from build123d import *

# Parameters (mm, degrees)
F1_DEPTH = 6.35
F2_R     = 5.08
F3_R     = 2.54
F4_R     = 2.54


with BuildPart() as f1:
    # F0 (on Top) → F1 (new body)
    with BuildSketch(Plane.XY):
        with BuildLine():
            Line((8.920526, 4.445), (10.377061, 4.445))
            ThreePointArc((10.377061, 4.445), (-11.288995, 0), (10.377061, -4.445))
            Line((10.377061, -4.445), (8.920526, -4.445))
            Line((8.920526, -4.445), (8.920526, 4.445))
        make_face()
        Polygon((3.739498, -6.477), (-3.739498, -6.477), (-7.478995, 0), (-3.739498, 6.477), (3.739498, 6.477), (7.478995, 0), align=None, mode=Mode.SUBTRACT)
        with BuildLine():
            ThreePointArc((10.377061, -4.445), (11.058662, -2.268791), (11.288995, 0))
            ThreePointArc((11.288995, 0), (11.058662, 2.268791), (10.377061, 4.445))
            Line((10.377061, 4.445), (8.920526, 4.445))
            Line((8.920526, 4.445), (8.920526, -4.445))
            Line((8.920526, -4.445), (10.377061, -4.445))
        make_face()
        with BuildLine():
            ThreePointArc((10.377061, 4.445), (11.058662, 2.268791), (11.288995, 0))
            ThreePointArc((11.288995, 0), (11.058662, -2.268791), (10.377061, -4.445))
            Line((10.377061, -4.445), (72.420526, -4.445))
            Line((72.420526, -4.445), (72.420526, 4.445))
            Line((72.420526, 4.445), (10.377061, 4.445))
        make_face()
    extrude(amount=F1_DEPTH)

    # F2
    f2_edges = [f1.edges().sort_by_distance(p)[0] for p in [
        (10.377061, -4.445, 3.175),
        (10.377061, 4.445, 3.175),
    ]]
    fillet(f2_edges, radius=F2_R)

    # F3
    f3_edges = [f1.edges().sort_by_distance(p)[0] for p in [
        (72.420526, 4.445, 3.175),
        (72.420526, -4.445, 3.175),
    ]]
    fillet(f3_edges, radius=F3_R)

    # F4
    f4_edges = [f1.edges().sort_by_distance(p)[0] for p in [
        (41.596433, -4.445, 6.35),
    ]]
    fillet(f4_edges, radius=F4_R)


solid = f1.part
The listing builds one solid part. Answer for the finished solid, in the listing's coordinates (mm). A direction names the side the tool comes from. Coordinates: 2 decimals unless noted, no trailing zeros. Order: outer loops, then holes, each group sorted by start corner. A loop starts at its lowest first (then second) coordinate and runs counter-clockwise, first axis right, second up.
Q1. A cutting plane is placed at B-B, the plane x = 22. Write down the section's boundary in (y, z) (3 decimals).
Q2. Which of the six approach directions +Z, -Z, +X, -X, +Y, -Y give full straight-line access (tool end or side, diameter ignored) to faces 5 (the face through (41.2, 3.721, 5.586)), 6 (the face through (41, -4.445, 2)), 7 (the face through (11, 5, 2)), 8 (the face through (5.583, 3.284, 3.131))?
Q3. A cutting plane is placed at A-A, the plane z = 2. Write down the section's boundary in (x, y) (1 decimal).
Q4. For a pull along X with two mould halves and no side action, classify faces 1 (the face through (41.992, -3.721, 5.586)), 2 (the face through (71.696, 0.027, 5.586)), 3 (the face through (5.635, -3.193, 3.131)), 4 (the face through (-11.28, 0.4, 1.88)) as pulls with the +X half, pulls with the -X half, needs draft (parallel to the pull), parting line crosses it, or undercut.
Q5. Given P1, Ø1.5, axis at x = 51, z = 3.5, coming from the +Y side (3 decimals); P2, Ø3, axis at y = 3.5, z = 5.5, coming from the +X side; P3, Ø12, axis at x = 17, y = 8.5, coming from the +Z side, each flat-ended and moving along its own axis, determine where each tip first touches the part or whether it passes through.
Q6. Consider line 1 (Y direction, x = 39, z = 0.5) (3 decimals); line 2 (X direction, y = 5, z = 2); line 3 (X direction, y = -3, z = 2.75). Determine where each line is inside the solid, lowest interval first.
Answers follow:
1. outline: (-4.445, 0) - (4.445, 0) - (4.445, 3.81) arc R2.54 ccw to (1.905, 6.35) - (-1.905, 6.35) arc R2.54 ccw to (-4.445, 3.81) - close
2. face 5: +Z, +X, +Y
2. face 6: +Z, -Z, +X, -Y
2. face 7: +Z, -Z, +X, +Y
2. face 8: +Z, -Z
3. outline: (9.2, -6.6) arc R5.1 cw to (13.3, -4.4) - (69.9, -4.4) arc R2.5 ccw to (72.4, -1.9) - (72.4, 1.9) arc R2.5 ccw to (69.9, 4.4) - (13.3, 4.4) arc R5.1 cw to (9.2, 6.6) arc R11.3 ccw (long way) to start; hole (-7.5, 0) - (-3.7, -6.5) - (3.7, -6.5) - (7.5, 0) - (3.7, 6.5) - (-3.7, 6.5) - close
4. face 1: needs draft
4. face 2: pulls with the +X half
4. face 3: undercut
4. face 4: parting line crosses it
5. P1: stops at y = 4.445
5. P2: stops at x = 72.28
5. P3: stops at z = 6.28
6. line 1: y = -4.445 to 4.445
6. line 2: x = -10.12 to -4.59, 4.59 to 11
6. line 3: x = -10.88 to -5.75, 5.75 to 72.17
